Source: CAD feature listing. Evaluate the final solid. Frame: model axes, mm. A direction names the side the tool comes from. Round coordinates to 2 decimals unless told otherwise and drop trailing zeros. Loops run counter-clockwise (first coordinate to the right, second up) from the corner with the lowest first, then second, coordinate; pieces in that order, holes last.
Item 1: Section query C-C on y = 9.25. Return loops of the section in (x, z), then the cut area to 3 significant figures.
Item 2: Section query B-B on x = 0. Return loops of the section in (y, z).
Item 3: Access query for faces 1 (the flat face through (3, 2.54, 11)), 2 (the cylindrical face through (12.242, 1.288, -12.265)), 3 (the cylindrical face through (0.29, 5.03, 8.23)). Directions: +Z, -Z, +X, -X, +Y, -Y. A direction counts if a zero-diameter tool reaches every point of the face in a straight line with its end or side. Return the directions, or none.
Item 4: Pull-direction query (Z, two-part tool) for faces 4 (the cylindrical face through (-7.61, 7.07, 5.83)), 5 (the cylindrical face through (-11.08, 1.25, 9.03)), 6 (the flat face through (12.7, 1, 0)); classes: released by +Z, released by -Z, zero draft, split by the parting line, or undercut.
Item 5: Ray query, L1, parallel to Z at x = 10.25, y = 2.5; L2, parallel to Z at x = 9.25, y = 2; L3, parallel to Y at x = 0, z = 8.6. Return the intervals inside material, ascending.
Item 6: Section query D-D on y = 6.35. Return loops of the section in (x, z), then the cut area to 3 significant figures.
Item 7: Section query A-A on z = 0. Return loops of the section in (x, y).
Item 8: First-contact query: P1, Ø3.5, axis at x = 0, y = 6.35, coming from the -Z side; P2, Ø5, axis at x = -9.525, z = -9.525, coming from the +Y side; P3, Ø1, axis at y = 8.5, z = -7, coming from the -X side; P4, Ø8.5, axis at x = 0, z = 0, coming from the +Y side (3 decimals). Flat tips, straight axial feed; report the tip coordinate or a pass-through.
```python
from build123d import *

# Parameters (mm, degrees)
SKETCH1_W                     = 25.4
SKETCH1_H                     = 25.4
BOSS_EXTRUDE1_DEPTH           = 2.54
SKETCH2_R                     = 9.5885
SKETCH2_R_2                   = 7.0485
EXTRUDE_THIN1_DEPTH           = 7.62
TAP_DRILL_FOR_6_32_TAP1_D     = 2.7051
TAP_DRILL_FOR_6_32_TAP1_DEPTH = 12.7
TAP_DRILL_FOR_6_32_TAP1_TIP   = 0.81269403
FILLET1_R                     = 1.524
FILLET2_R                     = 1.524
CUT_EXTRUDE1_START            = -7.62
SKETCH2_2_R                   = 7.0485
CUT_EXTRUDE1_DEPTH            = 7.62
FILLET3_R                     = 0.508
F_4_CLEARANCE_HOLE4_D         = 3.2639
F_4_CLEARANCE_HOLE4_DEPTH     = 2.54
F_4_CLEARANCE_HOLE4_TIP       = 0.980574487


with BuildPart() as part:
    # Sketch1 → Boss-Extrude1 (new body)
    with BuildSketch(Plane(origin=(0, 0, 0), x_dir=(1, 0, 0), z_dir=(0, 1, 0))):
        Rectangle(SKETCH1_W, SKETCH1_H)
    extrude(amount=BOSS_EXTRUDE1_DEPTH)

    # Sketch2 → Extrude-Thin1 (add)
    with BuildSketch(Plane(origin=(0, 2.54, 0), x_dir=(1, 0, 0), z_dir=(0, 1, 0))):
        Circle(SKETCH2_R)
        Circle(SKETCH2_R_2, mode=Mode.SUBTRACT)
    extrude(amount=EXTRUDE_THIN1_DEPTH)

    # Tap Drill for _6-32 Tap1
    with Locations(Plane.XY.offset(12.7)):
        with Locations((0, 6.35)):
            Hole(TAP_DRILL_FOR_6_32_TAP1_D / 2, depth=TAP_DRILL_FOR_6_32_TAP1_DEPTH)
            with Locations((0, 0, -(TAP_DRILL_FOR_6_32_TAP1_DEPTH + TAP_DRILL_FOR_6_32_TAP1_TIP / 2))):  # 118° drill point
                Cone(0, TAP_DRILL_FOR_6_32_TAP1_D / 2, TAP_DRILL_FOR_6_32_TAP1_TIP, mode=Mode.SUBTRACT)

    # Fillet1
    fillet1_edges = [part.edges().sort_by_distance(p)[0] for p in [
        (-9.5885, 2.54, 0),
    ]]
    fillet(fillet1_edges, radius=FILLET1_R)

    # Fillet2
    fillet2_edges = [part.edges().sort_by_distance(p)[0] for p in [
        (-12.7, 1.27, -12.7),
        (12.7, 1.27, -12.7),
        (12.7, 1.27, 12.7),
        (-12.7, 1.27, 12.7),
    ]]
    fillet(fillet2_edges, radius=FILLET2_R)

    # Sketch2_2 → Cut-Extrude1 (cut)
    with BuildSketch(Plane(origin=(0, 2.54, 0), x_dir=(1, 0, 0), z_dir=(0, 1, 0)).offset(CUT_EXTRUDE1_START)):
        with Locations(Location((0, 0, 0), (0, 0, 270))):
            Circle(SKETCH2_2_R)
    extrude(amount=CUT_EXTRUDE1_DEPTH, mode=Mode.SUBTRACT)

    # Fillet3
    fillet3_edges = [part.edges().sort_by_distance(p)[0] for p in [
        (-7.0485, 10.16, 0),
        (0, 0, -7.0485),
    ]]
    fillet(fillet3_edges, radius=FILLET3_R)

    # 4 Clearance Hole4
    with Locations(Plane(origin=(0, 2.54, 0), x_dir=(1, 0, 0), z_dir=(0, 1, 0))):
        with Locations((9.525, 9.525), (9.525, -9.525), (-9.525, -9.525), (-9.525, 9.525)):
            Hole(F_4_CLEARANCE_HOLE4_D / 2, depth=F_4_CLEARANCE_HOLE4_DEPTH)
            with Locations((0, 0, -(F_4_CLEARANCE_HOLE4_DEPTH + F_4_CLEARANCE_HOLE4_TIP / 2))):  # 118° drill point
                Cone(0, F_4_CLEARANCE_HOLE4_D / 2, F_4_CLEARANCE_HOLE4_TIP, mode=Mode.SUBTRACT)


solid = part.part
```
Data:
1. outline: circle Ø19.18 at (0, 0); hole circle Ø14.1 at (0, 0)
1. area: 133 mm2
2. outline: (0, -12.7) - (2.54, -12.7) - (2.54, -11.11) arc R1.52 cw to (4.06, -9.59) - (10.16, -9.59) - (10.16, -7.56) arc R0.51 ccw to (9.65, -7.05) - (0.51, -7.05) arc R0.51 ccw to (0, -7.56) - close; (0, 7.56) arc R0.51 ccw to (0.51, 7.05) - (5, 7.05) - (5, 9.59) - (4.06, 9.59) arc R1.52 cw to (2.54, 11.11) - (2.54, 12.7) - (0, 12.7) - close; (7.7, 7.05) - (9.65, 7.05) arc R0.51 ccw to (10.16, 7.56) - (10.16, 9.59) - (7.7, 9.59) - close
3. face 1: +Y
3. face 2: -Z, +X, +Y, -Y
3. face 3: +Z
4. face 4: split by the parting line
4. face 5: undercut
4. face 6: zero draft
5. L1: z = -12.7 to -10.99, -8.06 to 8.06, 10.99 to 12.7
5. L2: z = -12.7 to -11.13, -7.92 to 7.92, 11.13 to 12.7
5. L3: y = 0 to 5, 7.7 to 10.16
6. outline: (-1.35, 6.92) - (-1.35, 9.49) arc R9.59 ccw (long way) to (1.35, 9.49) - (1.35, 6.92) arc R7.05 cw (long way) to start
6. area: 126 mm2
7. outline: (-12.7, 0) - (-7.56, 0) arc R0.51 ccw to (-7.05, 0.51) - (-7.05, 9.65) arc R0.51 ccw to (-7.56, 10.16) - (-9.59, 10.16) - (-9.59, 4.06) arc R1.52 cw to (-11.11, 2.54) - (-12.7, 2.54) - close; (7.05, 0.51) arc R0.51 ccw to (7.56, 0) - (12.7, 0) - (12.7, 2.54) - (11.11, 2.54) arc R1.52 cw to (9.59, 4.06) - (9.59, 10.16) - (7.56, 10.16) arc R0.51 ccw to (7.05, 9.65) - close
8. P1: stops at z = -9.59
8. P2: stops at y = 2.55
8. P3: stops at x = -7.05
8. P4: passes through
